Source: CAD feature listing. Evaluate the final solid. Frame: model axes, mm. A direction names the side the tool comes from. Coordinates: 2 decimals unless noted, no trailing zeros. Order: outer loops, then holes, each group sorted by start corner. A loop starts at its lowest first (then second) coordinate and runs counter-clockwise, first axis right, second up. Notation, with made-up numbers: (70, 37.5) -> (125, 37.5) arc R23 ccw to (125, 57.5) -> close; hole circle Ø3 at (-23.75, -13). An arc over 180 degrees is marked (long way). Put each result on its own line as item: value.
from build123d import *

# Parameters (mm, degrees)
SKETCH1_W          = 889
SKETCH1_H          = 31.75
EXTRUDE1_DEPTH     = 28.575
EXTRUDE2_REACH     = 891
SKETCH2_W          = 25.4
SKETCH2_H          = 25.4
HOLE1_D            = 6.35
HOLE1_DEPTH        = 3.175
LPATTERN1_COUNT    = 35
LPATTERN1_PITCH    = 25.4
HOLE2_D            = 9.652
HOLE2_DEPTH        = 3.175
LPATTERN2_COUNT    = 12
LPATTERN2_PITCH    = 25.4
HOLE3_D            = 9.652
HOLE3_DEPTH        = 3.175
HOLE4_D            = 9.652
HOLE4_DEPTH        = 3.175
LPATTERN3_COUNT    = 12
LPATTERN3_PITCH    = 25.4
HOLE5_D            = 3.175
HOLE5_DEPTH        = 3.175
HOLE6_D            = 6.35
HOLE6_DEPTH        = 3.175
LPATTERN4_COUNT    = 35
LPATTERN4_PITCH    = 25.4
FILLET1_R          = 3.175
FILLET2_R          = 3.175
FILLET3_R          = 6.35
FILLET4_R          = 6.35
SKETCH15_W         = 596.207849475
SKETCH15_H         = 40.608240695
CUT_EXTRUDE1_DEPTH = 77


with BuildPart() as part:
    # Sketch1 → Extrude1 (new body)
    with BuildSketch(Plane.XY.offset(3.175)):
        with Locations((428.480011997, 8.672957166)):
            Rectangle(SKETCH1_W, SKETCH1_H)
    extrude(amount=-EXTRUDE1_DEPTH)

    # Sketch2 → Extrude2 (cut, up to next)
    with BuildSketch(Plane.ZY.offset(16.019988003), mode=Mode.PRIVATE) as extrude2_sk1:
        with Locations((-12.7, 8.672957166)):
            Rectangle(SKETCH2_W, SKETCH2_H)
    extrude2_tool1 = extrude(extrude2_sk1.sketch, amount=-EXTRUDE2_REACH, mode=Mode.PRIVATE) & part.part
    add(extrude2_tool1.solids().sort_by_distance((-16.019988, 8.672957, -12.7))[0], mode=Mode.SUBTRACT)

    # Hole1
    with Locations(Plane(origin=(0, 24.547957166, 0), x_dir=(-1, 0, 0), z_dir=(0, 1, 0))):
        with Locations((3.319988003, -12.7)):
            hole1 = Hole(HOLE1_D / 2, depth=HOLE1_DEPTH)

    # LPattern1: Hole1 ×35
    with Locations(*[(i * LPATTERN1_PITCH, 0, 0) for i in range(1, LPATTERN1_COUNT)]):
        add(hole1, mode=Mode.SUBTRACT)

    # Hole2
    with Locations(Plane.XY.offset(3.175)):
        with Locations((66.530011997, 10.577957166)):
            hole2 = Hole(HOLE2_D / 2, depth=HOLE2_DEPTH)

    # LPattern2: Hole2 ×12, 8 skipped
    with Locations(*[(i * LPATTERN2_PITCH, 0, 0) for i in range(1, LPATTERN2_COUNT) if i not in (2, 3, 4, 5, 6, 7, 8, 9)]):
        add(hole2, mode=Mode.SUBTRACT)

    # Hole3
    with Locations(Plane.XY.offset(3.175)):
        with Locations((428.480011997, 6.767957166)):
            Hole(HOLE3_D / 2, depth=HOLE3_DEPTH)

    # Hole4
    with Locations(Plane.XY.offset(3.175)):
        with Locations((511.030011997, 10.577957166)):
            hole4 = Hole(HOLE4_D / 2, depth=HOLE4_DEPTH)

    # LPattern3: Hole4 ×12, 8 skipped
    with Locations(*[(i * LPATTERN3_PITCH, 0, 0) for i in range(1, LPATTERN3_COUNT) if i not in (2, 3, 4, 5, 6, 7, 8, 9)]):
        add(hole4, mode=Mode.SUBTRACT)

    # Hole5
    with Locations(Plane.XY.offset(3.175)):
        with Locations((669.780011997, 8.672957166)):
            Hole(HOLE5_D / 2, depth=HOLE5_DEPTH)

    # Hole6
    with Locations(Plane(origin=(0, -4.027042834, 0), x_dir=(-1, 0, 0), z_dir=(0, 1, 0))):
        with Locations((3.319988003, -12.7)):
            hole6 = Hole(HOLE6_D / 2, depth=HOLE6_DEPTH)

    # LPattern4: Hole6 ×35
    with Locations(*[(i * LPATTERN4_PITCH, 0, 0) for i in range(1, LPATTERN4_COUNT)]):
        add(hole6, mode=Mode.SUBTRACT)

    # Fillet1
    fillet1_edges = [part.edges().sort_by_distance(p)[0] for p in [
        (428.480011997, 21.372957166, 0),
    ]]
    fillet(fillet1_edges, radius=FILLET1_R)

    # Fillet2
    fillet2_edges = [part.edges().sort_by_distance(p)[0] for p in [
        (428.480011997, -4.027042834, 0),
    ]]
    fillet(fillet2_edges, radius=FILLET2_R)

    # Fillet3
    fillet3_edges = [part.edges().sort_by_distance(p)[0] for p in [
        (428.480011997, -7.202042834, 3.175),
    ]]
    fillet(fillet3_edges, radius=FILLET3_R)

    # Fillet4
    fillet4_edges = [part.edges().sort_by_distance(p)[0] for p in [
        (428.480011997, 24.547957166, 3.175),
    ]]
    fillet(fillet4_edges, radius=FILLET4_R)

    # Sketch15 → Cut-Extrude1 (cut)
    with BuildSketch(Plane(origin=(0, 24.547957166, 0), x_dir=(1, 0, 0), z_dir=(0, 1, 0))):
        with Locations((582.083936734, 5.095879653)):
            Rectangle(SKETCH15_W, SKETCH15_H)
    extrude(amount=-CUT_EXTRUDE1_DEPTH, mode=Mode.SUBTRACT)


solid = part.part
1. Cut plane B-B on z = -12.7. Count the separate pieces of the cut face and the enclosed holes in it, plus the area to 3 significant figures.
Numbers:
separate pieces: 26
enclosed holes: 0
area: 1,420 mm2
2. First-contact query: pin 1 (7.5 mm diameter, centred on x = 174.48, z = -12.7, fed in from -Y); pin 2 (12.5 mm diameter, centred on x = 91.93, y = 10.58, fed in from -Z). Flat tips, straight axial feed; report the tip coordinate or a pass-through.
Numbers:
pin 1: stops at y = -7.2
pin 2: stops at z = 0
3. Set-up query: faces 1 (the flat face through (132, -4.027, -14)), 2 (the cylindrical face through (136.1, 22.6, 1.4)). Return all of +Z, -Z, +X, -X, +Y, -Y with unobstructed straight access to the full face (end or side cutting, diameter ignored); none if empty.
Numbers:
face 1: -Z, +X, -X
face 2: +Z, +X, -X, +Y
4. Cut plane A-A on x = 241.5. Output: boundary loops of the cut face in (y, z) (3 decimals).
Numbers:
outline: (-7.202, -25.4) -> (-4.027, -25.4) -> (-4.027, -3.175) arc R3.175 cw to (-0.852, 0) -> (18.198, 0) arc R3.175 cw to (21.373, -3.175) -> (21.373, -25.4) -> (24.548, -25.4) -> (24.548, -3.175) arc R6.35 ccw to (18.198, 3.175) -> (-0.852, 3.175) arc R6.35 ccw to (-7.202, -3.175) -> close
5. Ray query, line 1 along Y through (x, z) = (43, -15.75); line 2 along Z through (x, y) = (182.5, 15.5) (3 decimals); line 3 along Y through (x, z) = (141, -0.5). Return the intervals inside material, ascending.
Numbers:
line 1: y = -7.2 to -4.03, 21.37 to 24.55
line 2: z = 0 to 3.175
line 3: y = -6.61 to -2.56, 19.91 to 23.96
6. Pull-direction query (Y, two-part tool) for faces 3 (the flat face through (132, 24.548, -14)), 4 (the cylindrical face through (75.91, -5.64, -11.75)), 5 (the cylindrical face through (87.327, 12.028, 1.565)), 6 (the cylindrical face through (136.08, -5.391, 1.265)); classes: pulls with the +Y half, pulls with the -Y half, needs draft (parallel to the pull), parting line crosses it, or undercut.
Numbers:
face 3: pulls with the +Y half
face 4: needs draft
face 5: undercut
face 6: pulls with the -Y half
